from build123d import *

# Parameters (mm, degrees)
F0_R      = 8.2136813159
F0_R_2    = 8.2169
F1_DEPTH  = 19.304
F2_W      = 42.0680484259
F2_H      = 48.3717918396
F3_DEPTH  = 34.29
F4_DEPTH  = 5.588
F5_DEPTH  = 5.588
F8_DEPTH  = 34.29
F9_DEPTH  = 60.198
F10_R     = 3.577492803
F11_DEPTH = 65.786


# Not quite as in the source:
# - a feature names something its author has since deleted; it is built from what else it names


with BuildPart() as f1:
    # F0 (on Top) → F1 (new body)
    with BuildSketch(Plane.XY):
        with BuildLine():
            Line((25.4, -38.1), (25.4, 38.1))
            ThreePointArc((25.4, 38.1), (0, 12.7), (-25.4, 38.1))
            Line((-25.4, 38.1), (-25.4, -38.1))
            ThreePointArc((-25.4, -38.1), (0, -12.7), (25.4, -38.1))
        make_face()
        with BuildLine():
            ThreePointArc((-25.4, -38.1), (0, -63.5), (25.4, -38.1))
            ThreePointArc((25.4, -38.1), (0, -12.7), (-25.4, -38.1))
        make_face()
        with Locations((0, -38.1)):
            Circle(F0_R, mode=Mode.SUBTRACT)
        with BuildLine():
            ThreePointArc((-25.4, 38.1), (0, 12.7), (25.4, 38.1))
            ThreePointArc((25.4, 38.1), (0, 63.5), (-25.4, 38.1))
        make_face()
        with Locations((0, 38.1)):
            Circle(F0_R_2, mode=Mode.SUBTRACT)
    extrude(amount=F1_DEPTH)

    # F2 (on face) → F3 (join)
    with BuildSketch(Plane.XY.offset(19.304)):
        with Locations((-0.0028242129, -0.8024219424)):
            Rectangle(F2_W, F2_H)
    extrude(amount=F3_DEPTH)

    # F4 (cut): a face of the model
    f4_faces = [f1.faces().sort_by_distance(p)[0] for p in [
        (21.0312, -0.8024219424, 36.449),
    ]]
    extrude(f4_faces, amount=-F4_DEPTH, mode=Mode.SUBTRACT)

    # F5 (cut): a face of the model
    f5_faces = [f1.faces().sort_by_distance(p)[0] for p in [
        (-21.0368484259, -0.8024219424, 36.449),
    ]]
    extrude(f5_faces, amount=-F5_DEPTH, mode=Mode.SUBTRACT)

    # F7 (on face) → F8 (cut)
    with BuildSketch(Plane.YZ.offset(15.4432)):
        with BuildLine():
            Line((12.8851897717, 53.594), (-13.8123355974, 53.594))
            Line((-13.8123355974, 53.594), (-13.8123355974, 34.4488508999))
            ThreePointArc((-13.8123355974, 34.4488508999), (-0.4635729128, 24.7413409198), (12.8851897717, 34.4488508999))
            Line((12.8851897717, 34.4488508999), (12.8851897717, 53.594))
        make_face()
    extrude(amount=-F8_DEPTH, mode=Mode.SUBTRACT)

    # F6 (on face) → F9 (cut)
    with BuildSketch(Plane.XZ.offset(24.9883178622)):
        with BuildLine():
            ThreePointArc((-15.4488484259, 45.4977191985), (0.2250638301, 53.5401239092), (15.4432, 44.6654334664))
            Line((15.4432, 44.6654334664), (15.4432, 53.594))
            Line((15.4432, 53.594), (-15.4488484259, 53.594))
            Line((-15.4488484259, 53.594), (-15.4488484259, 45.4977191985))
        make_face()
    extrude(amount=-F9_DEPTH, mode=Mode.SUBTRACT)

    # F10 (on face) → F11 (cut)
    with BuildSketch(Plane.XZ.offset(24.9883178622)):
        with Locations((0.2250638301, 43.7909998)):
            Circle(F10_R)
    extrude(amount=-F11_DEPTH, mode=Mode.SUBTRACT)


solid = f1.part
Read the model definition and answer for the solid it produces. Units are mm, in the model's axes. A direction names the side the tool comes from. Give positions to 0.01 mm unless a question says otherwise; leave off trailing zeros. Write each loop counter-clockwise with the first axis right and the second up, starting at its lowest first coordinate (ties: lowest second). Pieces come first, ordered by that corner, then holes. Notation, with made-up numbers: M 53,22 L 109,22 A11 cw 109,34 Z; hole C 38,59.25 d2. An arc over 180 degrees is marked long. One line per item, written item: value. Start each with the question number.
(1) Find section C-C (x = -5.5). Determine the outline of the cut face in (y, z), plus the area to 3 significant figures.
(2) Find the intervals of material crossed by line 1 (Y direction, x = 0, z = 8); line 2 (X direction, y = 38, z = 9); line 3 (Z direction, x = -16, y = -30.5), in increasing order.
(3) Determine the mould class of faces 1 (the cylindrical face through (-0.24, 18.06, 47.34)), 2 (the cylindrical face through (0.559, 63.494, 9.517)), 3 (the flat face through (0, 12.885, 40)) for opening direction Y: pulls with the +Y half, pulls with the -Y half, needs draft (parallel to the pull), parting line crosses it, or undercut.
(4) Flat-ended cylindrical pins translate along their axes: pin 1 Ø11.5 at (x, z) = (0.23, 43.79) entering from -Y; pin 2 Ø2 at (y, z) = (39.5, 6.5) entering from +X; pin 3 Ø12 at (x, z) = (-19, 38) entering from +Y; pin 4 Ø4 at (x, y) = (6.5, 41.5) entering from -Z. Find the tip coordinate at first contact, or state that the pin passes through.
(5) A tool of negligible diameter and unlimited length cuts with its end or side. For faces 4 (the flat face through (0, -13.812, 40)), 5 (the flat face through (0, -24.988, 36)), 6 (the flat face through (15.443, -1, 23)), 7 (the flat face through (-15.449, -1, 23)), 8 (the flat face through (0, 23.383, 36)), from which of +Z, -Z, +X, -X, +Y, -Y can it reach the whole face along a straight path? Write none if from no direction.
(6) Find section A-A (z = 4.5). Determine the outline of the cut face in (x, y).
(7) Find section B-B (z = 50). Determine the outline of the cut face in (x, y), plus the area to 3 significant figures.
(8) Find section D-D (x = 0). Determine the outline of the cut face in (y, z), plus the area to 3 significant figures.
Results below:
1. outline: M -62.9,0 L -44.2,0 L -44.2,19.3 L -62.9,19.3 Z; M -32,0 L 32,0 L 32,19.3 L 23.38,19.3 L 23.38,52.78 L 12.89,52.78 L 12.89,34.45 A14.03 cw -13.81,34.45 L -13.81,52.78 L -24.99,52.78 L -24.99,19.3 L -32,19.3 Z; M 44.2,0 L 62.9,0 L 62.9,19.3 L 44.2,19.3 Z
1. area: 2,900 mm^2
2. line 1: y = -63.5 to -46.31, -29.89 to 29.88, 46.32 to 63.5
2. line 2: x = -25.4 to -8.22, 8.22 to 25.4
2. line 3: z = 0 to 19.3
3. face 1: needs draft
3. face 2: pulls with the +Y half
3. face 3: undercut
4. pin 1: stops at y = -24.99
4. pin 2: stops at x = 25.4
4. pin 3: stops at y = 23.38
4. pin 4: stops at z = 0
5. face 4: +Z, +X, -X
5. face 5: +Z, +X, -X, -Y
5. face 6: +Z, +X, +Y, -Y
5. face 7: +Z, -X, +Y, -Y
5. face 8: +Z, +X, -X, +Y
6. outline: M -25.4,-38.1 A25.4 ccw 25.4,-38.1 L 25.4,38.1 A25.4 ccw -25.4,38.1 Z; hole C 0,38.1 d16.43; hole C 0,-38.1 d16.43
7. outline: M -11.11,-24.99 L 10.57,-24.99 L 10.57,-13.81 L -11.11,-13.81 Z; M -11.11,12.89 L 10.57,12.89 L 10.57,23.38 L -11.11,23.38 Z
7. area: 470 mm^2
8. outline: M -63.5,0 L -46.31,0 L -46.31,19.3 L -63.5,19.3 Z; M -29.89,0 L 29.88,0 L 29.88,19.3 L 23.38,19.3 L 23.38,40.22 L 12.89,40.22 L 12.89,34.45 A14.03 cw -13.81,34.45 L -13.81,40.22 L -24.99,40.22 L -24.99,19.3 L -29.89,19.3 Z; M -24.99,47.36 L -13.81,47.36 L -13.81,53.54 L -24.99,53.54 Z; M 12.89,47.36 L 23.38,47.36 L 23.38,53.54 L 12.89,53.54 Z; M 46.32,0 L 63.5,0 L 63.5,19.3 L 46.32,19.3 Z
8. area: 2,620 mm^2
